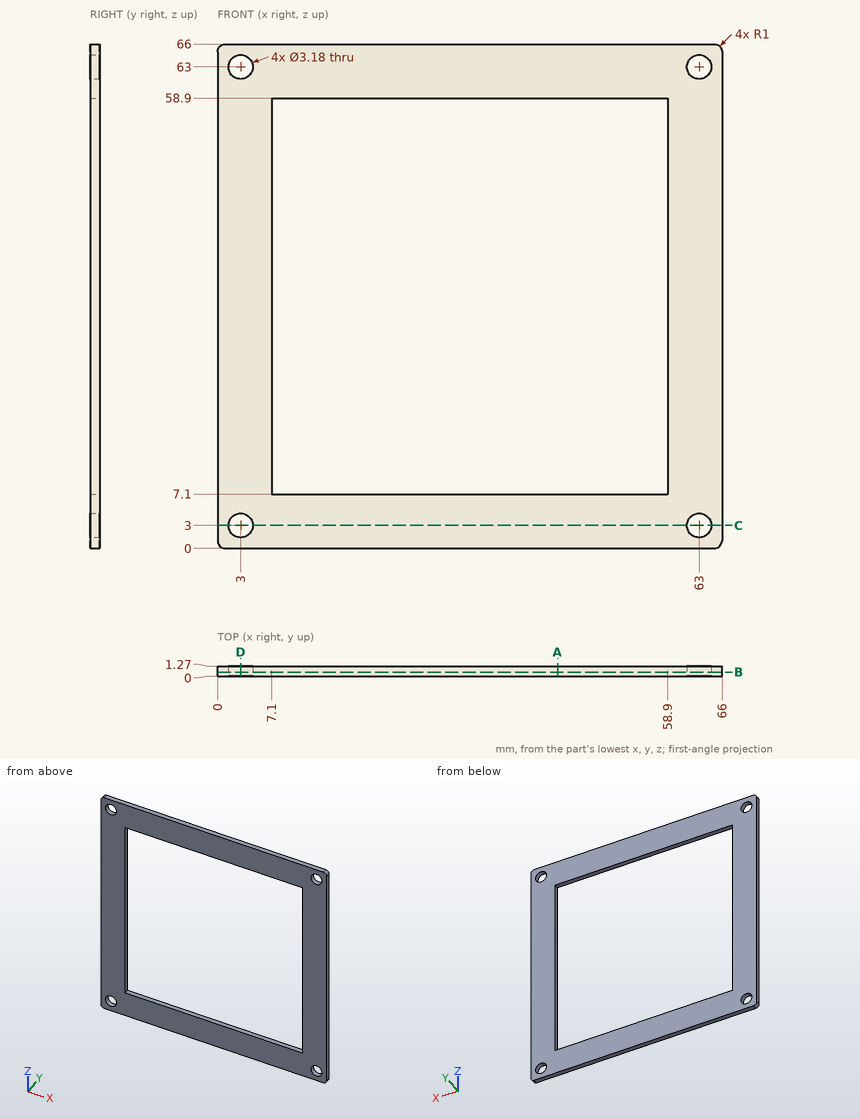
Input: dimensioned drawing with shaded views. Units: mm. Origin: part minimum x, y, z. Give positions to 0.01 mm unless a question says otherwise; leave off trailing zeros. Write each loop counter-clockwise with the first axis right and the second up, starting at its lowest first coordinate (ties: lowest second). Pieces come first, ordered by that corner, then holes. Notation, with made-up numbers: (48.25, 26) -> (97.25, 26) arc R23 ccw to (97.25, 59) -> close; hole circle Ø10 at (-31, -33). An arc over 180 degrees is marked (long way). Answer as a JSON object with one key per item and string values.
1. Cut plane B-B on y = 0.5. Output: boundary loops of the cut face in (x, z), and give its area (3 significant figures).
Ans:
{"outline": "(0, 1) arc R1 ccw to (1, 0) -> (65, 0) arc R1 ccw to (66, 1) -> (66, 65) arc R1 ccw to (65, 66) -> (1, 66) arc R1 ccw to (0, 65) -> close; hole circle Ø3.18 at (3, 3); hole circle Ø3.18 at (3, 63); hole (7.1, 7.1) -> (58.9, 7.1) -> (58.9, 58.9) -> (7.1, 58.9) -> close; hole circle Ø3.18 at (63, 3); hole circle Ø3.18 at (63, 63)", "area": "1,640 mm^2"}
2. Cut plane C-C on z = 3. Output: boundary loops of the cut face in (x, y).
Ans:
{"outline": "(0, 0) -> (1.41, 0) -> (1.41, 1.27) -> (0, 1.27) -> close; (4.59, 0) -> (61.41, 0) -> (61.41, 1.27) -> (4.59, 1.27) -> close; (64.59, 0) -> (66, 0) -> (66, 1.27) -> (64.59, 1.27) -> close"}
3. Cut plane D-D on x = 3. Output: boundary loops of the cut face in (y, z).
Ans:
{"outline": "(0, 0) -> (1.27, 0) -> (1.27, 1.41) -> (0, 1.41) -> close; (0, 4.59) -> (1.27, 4.59) -> (1.27, 61.41) -> (0, 61.41) -> close; (0, 64.59) -> (1.27, 64.59) -> (1.27, 66) -> (0, 66) -> close"}
4. Cut plane A-A on x = 44.5. Output: boundary loops of the cut face in (y, z).
Ans:
{"outline": "(0, 0) -> (1.27, 0) -> (1.27, 7.1) -> (0, 7.1) -> close; (0, 58.9) -> (1.27, 58.9) -> (1.27, 66) -> (0, 66) -> close"}
5. Ray query, probe 1 along X at (y, z) = (0.5, 63); probe 2 along X at (y, z) = (0.4, 33). Return the intervals inside material, ascending. Write a range as from..to.
Ans:
{"probe 1": "x = 0..1.41, 4.59..61.41, 64.59..66", "probe 2": "x = 0..7.1, 58.9..66"}
6. Contact query for flat-ended pins moving along their axis: pin 1 (2.5 mm diameter, centred on x = 3, z = 63, fed in from -Y); pin 2 (4 mm diameter, centred on x = 63, z = 63, fed in from -Y). Output: stop coordinate, or through.
Ans:
{"pin 1": "passes through", "pin 2": "stops at y = 0"}
